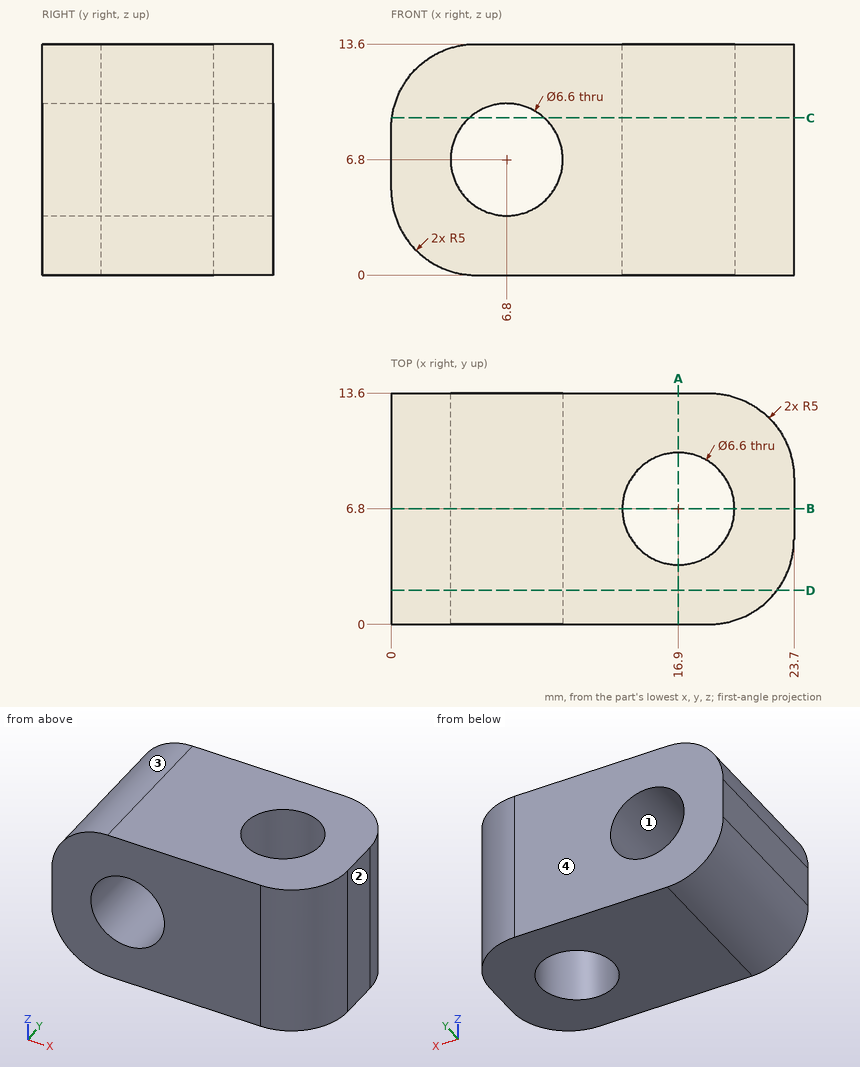
Study the drawing (mm; zero at the part's minimum x, y, z) and answer. Give positions to 0.01 mm unless a question says otherwise; leave off trailing zeros. Loops run counter-clockwise (first coordinate to the right, second up) from the corner with the lowest first, then second, coordinate; pieces in that order, holes last. Notation, with made-up numbers: (56.25, 69) - (91.25, 69) arc R31 cw to (91.25, 93) - close; hole circle Ø10 at (-31, 58). An arc over 180 degrees is marked (long way). Answer in a Markdown table with one row per item. Add a question column.
Q1. The part is cut by section C-C (z = 9.25). Determine the outline of the cut face in (x, y).
Q2. Consider line 1 along Z through (x, y) = (6.8, 3.25); line 2 along X through (y, z) = (6.25, 8.5); line 3 along X through (y, z) = (8.5, 9). Determine where each line is inside the solid, lowest interval first.
Q3. This flat-tipped pin is pushed along its axis until it touches: P1, Ø5.5, axis at x = 6.8, z = 6.8, coming from the -Y side. Where does it stop, or does it pass through?
Q4. The part is cut by section B-B (y = 6.8). Determine the outline of the cut face in (x, z).
Q5. Determine the mould class of the marked faces 1, 2, 3 and 4 for opening direction X: released by +X, released by -X, zero draft, split by the parting line, or undercut.
Q6. The part is cut by section D-D (y = 2). Determine the outline of the cut face in (x, z), and give its area (3 significant figures).
Q7. The part is cut by section A-A (x = 16.9). Determine the outline of the cut face in (y, z), and give its area (3 significant figures).
Solution:
| question | item | result |
|---|---|---|
| 1 | outline | (0.04, 0) - (4.59, 0) - (4.59, 13.6) - (0.04, 13.6) - close; (9.01, 0) - (18.7, 0) arc R5 ccw to (23.7, 5) - (23.7, 8.6) arc R5 ccw to (18.7, 13.6) - (9.01, 13.6) - close; hole circle Ø6.6 at (16.9, 6.8) |
| 2 | line 1 | z = 0 to 3.5, 10.1 to 13.6 |
| 2 | line 2 | x = 0 to 3.97, 9.63 to 13.65, 20.15 to 23.7 |
| 2 | line 3 | x = 0.02 to 4.34, 9.26 to 14.07, 19.73 to 23.7 |
| 3 | P1 | passes through |
| 4 | outline | (0, 5) arc R5 ccw to (5, 0) - (13.6, 0) - (13.6, 13.6) - (5, 13.6) arc R5 ccw to (0, 8.6) - close; (20.2, 0) - (23.7, 0) - (23.7, 13.6) - (20.2, 13.6) - close; hole circle Ø6.6 at (6.8, 6.8) |
| 5 | face 1 | undercut |
| 5 | face 2 | released by +X |
| 5 | face 3 | released by -X |
| 5 | face 4 | zero draft |
| 6 | outline | (0, 5) arc R5 ccw to (5, 0) - (22.7, 0) - (22.7, 13.6) - (5, 13.6) arc R5 ccw to (0, 8.6) - close; hole circle Ø6.6 at (6.8, 6.8) |
| 6 | area | 264 mm² |
| 7 | outline | (0, 0) - (3.5, 0) - (3.5, 13.6) - (0, 13.6) - close; (10.1, 0) - (13.6, 0) - (13.6, 13.6) - (10.1, 13.6) - close |
| 7 | area | 95.2 mm² |
